Here's how the part is built. I have some questions about the finished solid (model axes, mm). A direction names the side the tool comes from. Round coordinates to 2 decimals unless told otherwise and drop trailing zeros. Write each loop counter-clockwise with the first axis right and the second up, starting at its lowest first coordinate (ties: lowest second). Pieces come first, ordered by that corner, then holes. Notation, with made-up numbers: (-26, 18.25) - (25, 18.25) arc R26 cw to (25, 32.25) - close; hole circle Ø5 at (1.5, 27). An arc over 180 degrees is marked (long way). Use one line per item in the form item = value. Start each with the question number.
1. We'd pull the mould along X, two halves only. Please class faces 1 (the flat face through (-3.175, -11, -150)), 2 (the flat face through (14, 1, 0)), 3 (the cylindrical face through (35.93, 1.565, -35.056)): +X half, -X half, draft (parallel to the pull), parting line (faces both ways), or undercut.
2. I want a section at B-B, the plane z = -279.4. List the corners of the cut face in (x, y) for me (1 decimal).
3. I want a section at D-D, the plane x = 46.5. List the corners of the cut face in (y, z) for me (3 decimals).
4. Which directions (+Z, -Z, +X, -X, +Y, -Y) give clear straight access to the entire face, cutting with the end or side of a thin tool? Please do faces 4 (the flat face through (24, 3.175, -150)), 5 (the flat face through (0, -13, -155)).
5. I want a section at C-C, the plane z = -57. List the corners of the cut face in (x, y) for me (3 decimals), plus the area to 3 significant figures.
6. If I drill on line 1 along Z through (x, y) = (25.4, 2); line 2 along Y through (x, z) = (30.5, -188.5) (3 decimals); line 3 along X through (y, z) = (-17.25, -123.5) (3 decimals), over which ranges is the centre line in solid material (lowest first)?
7. I want a section at A-A, the plane x = 25.4. List the corners of the cut face in (y, z) for me (1 decimal), plus the area to 3 significant figures.
8. Will these pins go through, and if not, where does the flat tip stop? pin 1 (12 mm diameter, centred on x = 30, z = -105.5, fed in from -Y); pin 2 (12 mm diameter, centred on y = -11.5, z = -109.5, fed in from +X).
Autodesk Inventor part; units mm, degrees
ref_plane "YZ Plane" through (0, 0, 0) normal (1, 0, 0) x (0, 1, 0)
ref_plane "XZ Plane" through (0, 0, 0) normal (0, 1, 0) x (-1, 0, 0)
ref_plane "XY Plane" through (0, 0, 0) normal (0, 0, 1) x (1, 0, 0)
sketch "Sketch1" plane through (0, 0, 0) normal (0, 1, 0) x (-1, 0, 0)
  line L0 (0, 0) -> (-50.8, 0)
  line L1 (-50.8, 0) -> (-50.8, -304.8)
  line L2 (-50.8, -304.8) -> (0, -304.8)
  line L3 (0, -304.8) -> (0, 0)
  circle A0 centre (-25.4, -25.4) radius 14.2875
  circle A1 centre (-25.4, -279.4) radius 14.2875
  dimension "d0" = 304.8
  dimension "d1" = 50.8
  dimension "d2" = 25.4
  dimension "d3" = 25.4
  dimension "d4" = 25.4
  dimension "d5" = 25.4
  dimension "d6" = 28.575
  dimension "d7" = 28.575
extrude "Extrusion1" add sketch "Sketch1" along normal blind 3.175
sketch "Sketch2" plane through (0, 0, -304.8) normal (-1, 0, 0) x (0, 0, 1)
  line L0 (304.8, 3.175) -> (0, 3.175)
  line L1 (0, 3.175) -> (0, 0)
  line L2 (0, 0) -> (304.8, 0)
  line L3 (304.8, 0) -> (304.8, 3.175)
extrude "Extrusion2" add sketch "Sketch2" along normal blind 3.175
sketch "Sketch3" plane through (0, 0, 0) normal (0, -1, 0) x (1, 0, 0)
  line L0 (0, 0) -> (-3.175, 0)
  line L1 (-3.175, 0) -> (-3.175, -304.8)
  line L2 (-3.175, -304.8) -> (0, -304.8)
  line L3 (0, -304.8) -> (0, 0)
extrude "Extrusion3" add sketch "Sketch3" along normal blind 25.4
properties part number "chainguard" material "Aluminum 6061"
Model answer:
q1.face_1 = -X half
q1.face_2 = draft
q1.face_3 = undercut
q2.outline = (-3.2, -25.4) - (0, -25.4) - (0, 0) - (11.1, 0) - (11.1, 3.2) - (-3.2, 3.2) - close; (39.7, 0) - (50.8, 0) - (50.8, 3.2) - (39.7, 3.2) - close
q3.outline = (0, -304.8) - (3.175, -304.8) - (3.175, 0) - (0, 0) - close
q4.face_4 = +Z, -Z, +X, -X, +Y
q4.face_5 = +Z, -Z, +X, -Y
q5.outline = (-3.175, -25.4) - (0, -25.4) - (0, 0) - (50.8, 0) - (50.8, 3.175) - (-3.175, 3.175) - close
q5.area = 252 mm2
q6.line_1 = -304.8 to -293.69, -265.11 to -39.69, -11.11 to 0
q6.line_2 = 0 to 3.175
q6.line_3 = -3.175 to 0
q7.outline = (0, -304.8) - (3.2, -304.8) - (3.2, -293.7) - (0, -293.7) - close; (0, -265.1) - (3.2, -265.1) - (3.2, -39.7) - (0, -39.7) - close; (0, -11.1) - (3.2, -11.1) - (3.2, 0) - (0, 0) - close
q7.area = 786 mm2
q8.pin_1 = 0
q8.pin_2 = 0
